For this review, take the finished solid that the model builds, in its own axes (mm). Give positions to 0.01 mm unless a question says otherwise; leave off trailing zeros. Loops run counter-clockwise (first coordinate to the right, second up) from the corner with the lowest first, then second, coordinate; pieces in that order, holes last. Notation, with made-up numbers: (48.5, 43) -> (105.5, 43) arc R21 cw to (105.5, 80) -> close; hole circle Ø10 at (-30.75, 8). An arc over 180 degrees is marked (long way). One line per question, with ' | ' between items. Start each with the question number.
(1) Draft analysis for pull direction Y (two halves, no side actions). For faces 1 (the flat face through (2.358, 4.138, -0.556)), 2 (the cylindrical face through (0.861, -2.076, -0.556)), 3 (the flat face through (-4.762, 0, -1)), state which applies: +Y half, -Y half, draft (parallel to the pull), parting line (faces both ways), or undercut.
(2) Wall thickness on probe 1 along Y at (x, z) = (-0.25, 0.5); probe 2 along X at (y, z) = (0.25, -14.5); probe 3 along X at (y, z) = (-1, -6): over which ranges is each line inside the solid? List them lowest first.
(3) Consider section A-A (x = 0). Write out the cut boundary in (y, z).
(4) Consider section D-D (y = 4). Write out the cut boundary in (x, z).
(5) Insertion check: P1, Ø3, axis at x = -2.5, z = 21, coming from the +Y side; P2, Ø3, axis at x = -3, z = -10.5, coming from the +Y side; P3, Ø1, axis at x = -2, z = -21, coming from the -Y side. Each pin has a flat end and moves straight along its axis. Give the tip position at first contact, or say it passes through.
(6) Consider section B-B (y = 0). Write out the cut boundary in (x, z).
(7) Consider section C-C (z = 24.5). Write out the cut boundary in (x, y), and give its area (3 significant figures).
Autodesk Inventor part; units mm, degrees
ref_plane "YZ Plane" through (0, 0, 0) normal (1, 0, 0) x (0, 1, 0)
ref_plane "XZ Plane" through (0, 0, 0) normal (0, 1, 0) x (-1, 0, 0)
ref_plane "XY Plane" through (0, 0, 0) normal (0, 0, 1) x (1, 0, 0)
sketch "Sketch1" plane through (0, 0, 0) normal (0, 0, 1) x (1, 0, 0)
  line L0 (-4.7625, -2.7496) -> (-4.7625, 2.7496)
  line L1 (-4.7625, 2.7496) -> (0, 5.4993)
  line L2 (0, 5.4993) -> (4.7625, 2.7496)
  line L3 (4.7625, 2.7496) -> (4.7625, -2.7496)
  line L4 (4.7625, -2.7496) -> (0, -5.4993)
  line L5 (0, -5.4993) -> (-4.7625, -2.7496)
  point P0 (0, 0)
  point P1 (0, 0)
  dimension "Size" = 9.525
extrude "Extrusion1" add sketch "Sketch1" along normal mid plane 79.375
sketch "Sketch3" plane through (0, 0, 39.6875) normal (0, 0, 1) x (1, 0, 0)
  line L0 (-4.7625, 2.7496) -> (0, 5.4993) construction
  line L1 (0, 5.4993) -> (4.7625, 2.7496) construction
  line L2 (4.7625, 2.7496) -> (4.7625, -2.7496) construction
  line L3 (4.7625, -2.7496) -> (0, -5.4993) construction
  line L4 (0, -5.4993) -> (-4.7625, -2.7496) construction
  line L5 (-4.7625, -2.7496) -> (-4.7625, 2.7496) construction
  point P0 (0, 0)
hole "Hole1" at (0, 0, 39.6875) direction (0, 0, -1) diameter 4.4958 end through all
sketch "Sketch4" plane through (0, 0, 39.6875) normal (0, 0, 1) x (1, 0, 0)
  circle A0 centre (0, 0) radius 2.2479 construction
  line L0 (-4.7625, 2.7496) -> (0, 5.4993) construction
  line L1 (0, 5.4993) -> (4.7625, 2.7496) construction
  line L2 (4.7625, 2.7496) -> (4.7625, -2.7496) construction
  line L3 (4.7625, -2.7496) -> (0, -5.4993) construction
  line L4 (0, -5.4993) -> (-4.7625, -2.7496) construction
  line L5 (-4.7625, -2.7496) -> (-4.7625, 2.7496) construction
  circle A1 centre (0, 0) radius 5.1245
  circle A2 centre (0, 0) radius 8.89
  dimension "thunder" = 10.2489
  dimension "d16" = 17.78
extrude "Extrusion3" cut sketch "Sketch4" against normal through all
equation "\"bearing\" = 25.4"
properties part number "GP1-005" material "Aluminum 6061"
A:
1) face 1: +Y half | face 2: undercut | face 3: draft
2) probe 1: y = -5.12 to -2.23, 2.23 to 5.12 | probe 2: x = -4.76 to -2.23, 2.23 to 4.76 | probe 3: x = -4.76 to -2.01, 2.01 to 4.76
3) outline: (-5.12, -39.69) -> (-2.25, -39.69) -> (-2.25, 39.69) -> (-5.12, 39.69) -> close; (2.25, -39.69) -> (5.12, -39.69) -> (5.12, 39.69) -> (2.25, 39.69) -> close
4) outline: (-2.6, -39.69) -> (2.6, -39.69) -> (2.6, 39.69) -> (-2.6, 39.69) -> close
5) P1: stops at y = 4.92 | P2: stops at y = 4.63 | P3: stops at y = -4.63
6) outline: (-4.76, -39.69) -> (-2.25, -39.69) -> (-2.25, 39.69) -> (-4.76, 39.69) -> close; (2.25, -39.69) -> (4.76, -39.69) -> (4.76, 39.69) -> (2.25, 39.69) -> close
7) outline: (-4.76, -1.89) arc R5.12 ccw to (-4.02, -3.18) -> (-0.74, -5.07) arc R5.12 ccw to (0.74, -5.07) -> (4.02, -3.18) arc R5.12 ccw to (4.76, -1.89) -> (4.76, 1.89) arc R5.12 ccw to (4.02, 3.18) -> (0.74, 5.07) arc R5.12 ccw to (-0.74, 5.07) -> (-4.02, 3.18) arc R5.12 ccw to (-4.76, 1.89) -> close; hole circle Ø4.5 at (0, 0) | area: 61.1 mm^2
